Geometry: final body of the model. Coordinates: model frame, mm. Face numbers are marked on the shaded views. A direction names the side the tool comes from. Coordinates: 2 decimals unless noted, no trailing zeros. Write each loop counter-clockwise with the first axis right and the second up, starting at its lowest first coordinate (ties: lowest second). Pieces come first, ordered by that corner, then holes. Notation, with made-up numbers: (61, 73) - (79, 73) arc R22 cw to (79, 101) - close; hole circle Ø4 at (-34, 47). An arc over 180 degrees is marked (long way). Answer as a JSON object with one key per item and string values. Group by question number.
Item 1: Line query: line 1 along Y through (x, z) = (7.75, 0); line 2 along Z through (x, y) = (23, 0); line 3 along Y through (x, z) = (69.5, 0.5). Output: solid intervals per line, ascending. Write a range as from..to.
Item 2: Section A-A on y = 0. Return loops of the section in (x, z).
Item 3: Set-up query: the marked faces 1 and 2. Return all of +Z, -Z, +X, -X, +Y, -Y with unobstructed straight access to the full face (end or side cutting, diameter ignored); none if empty.
Item 4: Section B-B on z = 0. State how many separate pieces and enclosed holes the cut face has, and give its area (3 significant figures).
Item 5: Mould query, pull axis Y, two halves, no side actions, for the marked faces 3, 4 and 5. Classes: pulls with the +Y half, pulls with the -Y half, needs draft (parallel to the pull), parting line crosses it, or undercut.
Item 6: Section C-C on x = 31. Return loops of the section in (y, z).
Item 7: First-contact query: pin 1 Ø10 at (x, z) = (60, 5.5) entering from -Y; pin 2 Ø5 at (x, y) = (32.5, 9) entering from +Z; pin 3 Ø5.5 at (y, z) = (23.5, 0) entering from +X; pin 4 Ø2 at (x, z) = (65, 13.5) entering from -Y. Flat tips, straight axial feed; report the tip coordinate or a pass-through.
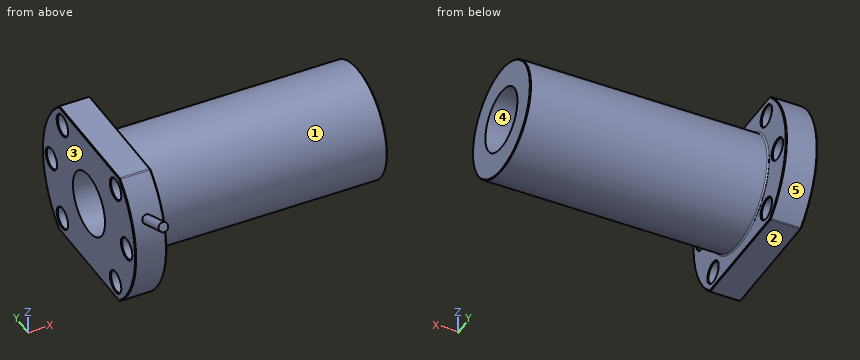
```python
from build123d import *

# Parameters (mm, degrees)
SKETCH_W        = 86
SKETCH_H        = 18
SKETCH001_R     = 29
PAD_DEPTH       = 10
SKETCH002_W     = 20
SKETCH002_H     = 49.824667
POCKET_DEPTH    = 86.001
SKETCH003_R     = 3.3
POCKET001_DEPTH = 86.001
SKETCH005_R     = 1.5
PAD001_DEPTH    = 29
FILLET_R        = 0.5
CHAMFER_SIZE    = 0.25
CHAMFER001_SIZE = 0.25
CHAMFER002_SIZE = 0.25
SKETCH007_R     = 10
POCKET002_DEPTH = 86.001


with BuildPart() as part:
    # Sketch → Revolution (revolve)
    with BuildSketch(Plane.XZ):
        with Locations((43, 9)):
            Rectangle(SKETCH_W, SKETCH_H)
    revolve(axis=Axis((0, 0, 0), (1, 0, 0)))

    # Sketch001 (on Face3 of Revolution) → Pad (new body)
    with BuildSketch(Plane(origin=(0, 0, 0), x_dir=(0, 0, -1), z_dir=(-1, 0, 0))):
        Circle(SKETCH001_R)
    extrude(amount=-PAD_DEPTH)

    # Sketch002 (on Face5 of Pad) → Pocket (cut, through all)
    with BuildSketch(Plane(origin=(0, 0, 0), x_dir=(0, 0, -1), z_dir=(-1, 0, 0))):
        with Locations((-32, 24.912333)):
            Rectangle(SKETCH002_W, SKETCH002_H)
        with Locations((-32, -24.912333)):
            Rectangle(SKETCH002_W, SKETCH002_H)
        with Locations((32, 24.912333)):
            Rectangle(SKETCH002_W, SKETCH002_H)
        with Locations((32, -24.912333)):
            Rectangle(SKETCH002_W, SKETCH002_H)
    extrude(amount=-POCKET_DEPTH, mode=Mode.SUBTRACT)

    # Sketch003 (on Face6 of Pocket) → Pocket001 (cut, through all)
    with BuildSketch(Plane(origin=(0, 0, 0), x_dir=(0, 0, -1), z_dir=(-1, 0, 0))):
        with Locations((-16.617001, -16.617018)):
            Circle(SKETCH003_R)
        with Locations((0, -23.5)):
            Circle(SKETCH003_R)
        with Locations((16.617012, -16.617007)):
            Circle(SKETCH003_R)
        with Locations((-16.617001, 16.617018)):
            Circle(SKETCH003_R)
        with Locations((0, 23.5)):
            Circle(SKETCH003_R)
        with Locations((16.617012, 16.617007)):
            Circle(SKETCH003_R)
    extrude(amount=-POCKET001_DEPTH, mode=Mode.SUBTRACT)

    # Sketch005 (on DatumPlane) → Pad001 (join)
    with BuildSketch(Plane(origin=(5, -36.955188, 15.307322), x_dir=(-1, 0, 0), z_dir=(0, 0.92388, -0.382683))):
        with Locations((0.138398, 0)):
            Circle(SKETCH005_R)
    extrude(amount=PAD001_DEPTH)

    # Fillet
    fillet_edges = [part.edges().sort_by_distance(p)[0] for p in [
        (10, 0, -18),
    ]]
    fillet(fillet_edges, radius=FILLET_R)

    # Chamfer
    chamfer_edges = [part.edges().sort_by_distance(p)[0] for p in [
        (0, 0, 22),
        (5, -18.894444, 22),
        (10, 0, 22),
        (5, 18.894444, 22),
        (0, -29, 0),
        (10, -29, 0),
        (0, 0, -22),
        (5, 18.894444, -22),
        (10, 0, -22),
        (5, -18.894444, -22),
        (0, 29, 0),
        (10, 29, 0),
    ]]
    chamfer(chamfer_edges, length=CHAMFER_SIZE)

    # Chamfer001
    chamfer001_edges = [part.edges().sort_by_distance(p)[0] for p in [
        (86, 0, -18),
    ]]
    chamfer(chamfer001_edges, length=CHAMFER001_SIZE)

    # Chamfer002
    chamfer002_edges = [part.edges().sort_by_distance(p)[0] for p in [
        (0, -16.617018, 19.917001),
        (5, -16.617018, 13.317001),
        (10, -16.617018, 19.917001),
        (0, 16.617018, 19.917001),
        (5, 16.617018, 13.317001),
        (10, 16.617018, 19.917001),
        (0, 23.5, 3.3),
        (5, 23.5, -3.3),
        (10, 23.5, 3.3),
        (0, 16.617007, -13.317012),
        (5, 16.617007, -19.917012),
        (10, 16.617007, -13.317012),
        (0, -23.5, 3.3),
        (5, -23.5, -3.3),
        (10, -23.5, 3.3),
        (0, -16.617007, -13.317012),
        (5, -16.617007, -19.917012),
        (10, -16.617007, -13.317012),
    ]]
    chamfer(chamfer002_edges, length=CHAMFER002_SIZE)

    # Sketch007 (on Face48 of Chamfer002) → Pocket002 (cut, through all)
    with BuildSketch(Plane(origin=(0, 0, 0), x_dir=(0, 0, -1), z_dir=(-1, 0, 0))):
        Circle(SKETCH007_R)
    extrude(amount=-POCKET002_DEPTH, mode=Mode.SUBTRACT)


solid = part.part
```
Checks:
{
 "1": {"line 1": "-29..-26.8, -20.2..-10, 10..20.2, 26.8..29", "line 2": "-18..-10, 10..18", "line 3": "-17.99..-9.99, 9.99..17.99"},
 "2": {"outline": "(0, -21.75) - (0.25, -22) - (9.75, -22) - (10, -21.75) - (10, -18.5) arc R0.5 cw to (10.5, -18) - (85.75, -18) - (86, -17.75) - (86, -10) - (0, -10) - close; (0, 10) - (86, 10) - (86, 17.75) - (85.75, 18) - (10.5, 18) arc R0.5 cw to (10, 18.5) - (10, 21.75) - (9.75, 22) - (0.25, 22) - (0, 21.75) - close"},
 "3": {"face 1": "+X", "face 2": "-Z, +X, -X, +Y, -Y"},
 "4": {"separate pieces": "4", "enclosed holes": "0", "area": "1,460 mm^2"},
 "5": {"face 3": "needs draft", "face 4": "undercut", "face 5": "pulls with the +Y half"},
 "6": {"outline": "circle Ø36 at (0, 0); hole circle Ø20 at (0, 0)"},
 "7": {"pin 1": "y = -17.99", "pin 2": "z = 16.79", "pin 3": "through", "pin 4": "y = -12.95"}
}
